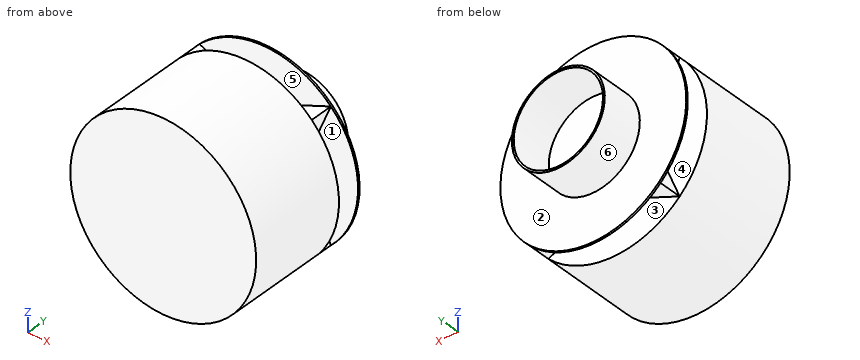
```python
from build123d import *

# Parameters (mm, degrees)
SKETCH11_R          = 304.8
BOSS_EXTRUDE5_DEPTH = 330.2
BOSS_EXTRUDE6_DEPTH = 76.2
SKETCH13_R          = 304.8
BOSS_EXTRUDE7_DEPTH = 6.096
SKETCH14_R          = 152.4
SKETCH14_R_2        = 146.304
BOSS_EXTRUDE8_DEPTH = 139.7


with BuildPart() as part:
    # Sketch11 → Boss-Extrude5 (new body)
    with BuildSketch(Plane(origin=(0, 0, 0), x_dir=(1, 0, 0), z_dir=(0, 1, 0))):
        with Locations(Location((0, 0, 0), (0, 0, 270))):
            Circle(SKETCH11_R)
    extrude(amount=BOSS_EXTRUDE5_DEPTH)

    # Sketch12 → Boss-Extrude6 (add)
    with BuildSketch(Plane(origin=(0, 330.2, 0), x_dir=(1, 0, 0), z_dir=(0, 1, 0))):
        Polygon((-127, 0), (-215.526146906, -215.526146906), (0, -127), (215.526146906, -215.526146906), (127, 0), (215.526146906, 215.526146906), (0, 127), (-215.526146906, 215.526146906), align=None)
    extrude(amount=BOSS_EXTRUDE6_DEPTH)

    # Sketch13 → Boss-Extrude7 (add)
    with BuildSketch(Plane(origin=(0, 406.4, 0), x_dir=(1, 0, 0), z_dir=(0, 1, 0))):
        with Locations(Location((0, 0, 0), (0, 0, 135))):
            Circle(SKETCH13_R)
    extrude(amount=BOSS_EXTRUDE7_DEPTH)

    # Sketch14 → Boss-Extrude8 (add)
    with BuildSketch(Plane(origin=(0, 412.496, 0), x_dir=(1, 0, 0), z_dir=(0, 1, 0))):
        with Locations(Location((0, 0, 0), (0, 0, 270))):
            Circle(SKETCH14_R)
        with Locations(Location((0, 0, 0), (0, 0, 270))):
            Circle(SKETCH14_R_2, mode=Mode.SUBTRACT)
    extrude(amount=BOSS_EXTRUDE8_DEPTH)


solid = part.part
```
Check sheet for the modelled part. Datum: model origin and axes. Units: mm. Face numbers are marked on the shaded views. A direction names the side the tool comes from. Round coordinates to 2 decimals unless told otherwise and drop trailing zeros. Loops run counter-clockwise (first coordinate to the right, second up) from the corner with the lowest first, then second, coordinate; pieces in that order, holes last. Notation, with made-up numbers: (0.25, 63.5) - (37.25, 63.5) arc R21 cw to (37.25, 99.5) - close; hole circle Ø10 at (75, -37). An arc over 180 degrees is marked (long way). Answer as a JSON object with one key per item and string values. Group by question number.
Q1. Sectioned sample at A-A, the plane y = 356. Enter the section's corners in (x, z).
Q2. Mould release check, pull along X, two halves, no side actions. Record for the marked faces 4, 5 and 6: released by +X, released by -X, zero draft, split by the parting line, or undercut.
Q3. Scan lines: line 1 along Y through (x, z) = (-138.5, -198); line 2 along X through (y, z) = (519, 0); line 3 along Y through (x, z) = (15.5, -113.5). Record each from-to range of solid material in increasing order. Write a range as [from, to].
Q4. Set-up check for the marked faces 1, 2 and 3: record each of +Z, -Z, +X, -X, +Y, -Y from which the full face is reachable in a straight line by a thin tool's end or side.
Q5. Sectioned sample at B-B, the plane x = 233. Enter the section's corners in (y, z), plus the area to 3 significant figures.
Q6. Gauge pin test, flat ends, axial feed: P1, Ø3, axis at x = 113, y = 125.5, coming from the +Z side; P2, Ø5, axis at x = 35.5, y = 216, coming from the +Z side; P3, Ø1, axis at x = -154, y = 90, coming from the -Z side; P4, Ø1.5, axis at x = 94.5, z = -225, coming from the -Y side. Record the tip position at first contact, or that the pin passes through.
Q7. Sectioned sample at D-D, the plane z = 30. Enter the section's corners in (x, y).
Q8. Sectioned sample at C-C, the plane y = 502. Enter the section's corners in (x, z).
Solution:
{
 "1": {"outline": "(-215.53, -215.53) - (0, -127) - (215.53, -215.53) - (127, 0) - (215.53, 215.53) - (0, 127) - (-215.53, 215.53) - (-127, 0) - close"},
 "2": {"face 4": "zero draft", "face 5": "undercut", "face 6": "split by the parting line"},
 "3": {"line 1": "y = [0, 330.2], [406.4, 412.5]", "line 2": "x = [-152.4, -146.3], [146.3, 152.4]", "line 3": "y = [0, 412.5]"},
 "4": {"face 1": "+X", "face 2": "+Y", "face 3": "-Z"},
 "5": {"outline": "(0, -196.5) - (330.2, -196.5) - (330.2, 196.5) - (0, 196.5) - close; (406.4, -196.5) - (412.5, -196.5) - (412.5, 196.5) - (406.4, 196.5) - close", "area": "132,000 mm²"},
 "6": {"P1": "stops at z = 283.67", "P2": "stops at z = 303.01", "P3": "stops at z = -263.33", "P4": "stops at y = 0"},
 "7": {"outline": "(-303.32, 0) - (303.32, 0) - (303.32, 330.2) - (139.32, 330.2) - (139.32, 406.4) - (303.32, 406.4) - (303.32, 412.5) - (149.42, 412.5) - (149.42, 552.2) - (143.2, 552.2) - (143.2, 412.5) - (-143.2, 412.5) - (-143.2, 552.2) - (-149.42, 552.2) - (-149.42, 412.5) - (-303.32, 412.5) - (-303.32, 406.4) - (-139.32, 406.4) - (-139.32, 330.2) - (-303.32, 330.2) - close"},
 "8": {"outline": "circle Ø304.8 at (0, 0); hole circle Ø292.61 at (0, 0)"}
}
